```python
from build123d import *

# Parameters (mm, degrees)
SKETCH_1_W          = 10
SKETCH_1_H          = 12
SKETCH_1_W_2        = 5.2
SKETCH_1_H_2        = 5.2
EXTRUDE_1_DEPTH     = 4
SKETCH_2_R          = 0.6
CUT_EXTRUDE_1_DEPTH = 13.328828006
SKETCH_3_R          = 0.7
CUT_EXTRUDE_2_DEPTH = 14.601470509
SKETCH_3_3_R        = 1
CUT_EXTRUDE_3_DEPTH = 1.4
CUT_EXTRUDE_START   = -10.6
SKETCH_3_4_R        = 1
CUT_EXTRUDE_4_DEPTH = 1.4


with BuildPart() as part:
    # 草图1 → 凸台-拉伸1 (new body)
    with BuildSketch(Plane(origin=(0, 0, 0), x_dir=(1, 0, 0), z_dir=(0, 1, 0))):
        Rectangle(SKETCH_1_W, SKETCH_1_H)
        Rectangle(SKETCH_1_W_2, SKETCH_1_H_2, mode=Mode.SUBTRACT)
    extrude(amount=EXTRUDE_1_DEPTH)

    # 草图2 → 切除-拉伸1 (cut, through all)
    with BuildSketch(Plane(origin=(5, 0, 0), x_dir=(0, 0, -1), z_dir=(1, 0, 0))):
        with Locations((0, 2)):
            Circle(SKETCH_2_R)
    extrude(amount=-CUT_EXTRUDE_1_DEPTH, mode=Mode.SUBTRACT)

    # 草图3 → 切除-拉伸2 (cut, through all)
    with BuildSketch(Plane(origin=(0, 0, -6), x_dir=(-1, 0, 0), z_dir=(0, 0, -1))):
        with Locations((0, 2)):
            Circle(SKETCH_3_R)
    extrude(amount=-CUT_EXTRUDE_2_DEPTH, mode=Mode.SUBTRACT)

    # 草图3<3> → 切除-拉伸3 (cut)
    with BuildSketch(Plane(origin=(0, 0, -6), x_dir=(-1, 0, 0), z_dir=(0, 0, -1))):
        with Locations((0, 2)):
            Circle(SKETCH_3_3_R)
    extrude(amount=-CUT_EXTRUDE_3_DEPTH, mode=Mode.SUBTRACT)

    # 草图3<4> → 切除-拉伸4 (cut)
    with BuildSketch(Plane(origin=(0, 0, -6), x_dir=(-1, 0, 0), z_dir=(0, 0, -1)).offset(CUT_EXTRUDE_START)):
        with Locations((0, 2)):
            Circle(SKETCH_3_4_R)
    extrude(amount=-CUT_EXTRUDE_4_DEPTH, mode=Mode.SUBTRACT)


solid = part.part
```
Geometry: final body of the model. Coordinates: model frame, mm. A direction names the side the tool comes from. Coordinates: 2 decimals unless noted, no trailing zeros. Order: outer loops, then holes, each group sorted by start corner. A loop starts at its lowest first (then second) coordinate and runs counter-clockwise, first axis right, second up. Notation, with made-up numbers: (-18, 45) - (26, 45) arc R10 cw to (26, 53) - close; hole circle Ø11 at (-32, 17). An arc over 180 degrees is marked (long way). Return JSON: item names as keys, results as strings. Group by question number.
1. Cut plane C-C (z = 2). Output: boundary loops of the cut face in (x, y).
2. Pull-direction query (X, two-part tool) for faces 6 (the face through (-1.2, 2, -6)), 7 (the face through (-5, 1, 0)), 8 (the face through (-2.6, 2, 1)); classes: pulls with the +X half, pulls with the -X half, needs draft (parallel to the pull), parting line crosses it, or undercut.
3. Cut plane B-B (x = 0). Output: boundary loops of the cut face in (y, z).
4. Pin query (flat end, axial travel): pin 1 (1.6 mm diameter, centred on x = 0, y = 2, fed in from -Z); pin 2 (6 mm diameter, centred on x = 0.5, z = -1, fed in from +Y); pin 3 (1 mm diameter, centred on y = 2, z = 0, fed in from +X); pin 4 (1.6 mm diameter, centred on x = 0, y = 2, fed in from +Z). Return the tip coordinate at first contact, or that it passes through.
5. Cut plane A-A (y = 2). Count the separate pieces of the cut face and the enclosed holes in it, plus the area to 3 significant figures.
6. Cut plane D-D (x = -1.25). Output: boundary loops of the cut face in (y, z), plus the area to 3 significant figures.
7. Material intervals for line 1 along X through (y, z) = (0.45, -0.75); line 2 along Z through (x, y) = (-2.25, 0.3); line 3 along Z through (x, y) = (-3.25, 2.15), sorted ascending. Write a range as [from, to].
8. Set-up query: faces 1 (the face through (-1, 2, 2.6)), 2 (the face through (0, 1, -5)), 3 (the face through (0, 4, -3)), 4 (the face through (0, 1, 5)), 5 (the face through (3.817, 2.506, -0.323)). Return all of +Z, -Z, +X, -X, +Y, -Y with unobstructed straight access to the full face (end or side cutting, diameter ignored); none if empty.
Resolved:
{
 "1": {"outline": "(-5, 0) - (-2.6, 0) - (-2.6, 4) - (-5, 4) - close; (2.6, 0) - (5, 0) - (5, 4) - (2.6, 4) - close"},
 "2": {"face 6": "needs draft", "face 7": "pulls with the -X half", "face 8": "undercut"},
 "3": {"outline": "(0, -6) - (1, -6) - (1, -4.6) - (1.3, -4.6) - (1.3, -2.6) - (0, -2.6) - close; (0, 2.6) - (1.3, 2.6) - (1.3, 4.6) - (1, 4.6) - (1, 6) - (0, 6) - close; (2.7, -4.6) - (3, -4.6) - (3, -6) - (4, -6) - (4, -2.6) - (2.7, -2.6) - close; (2.7, 2.6) - (4, 2.6) - (4, 6) - (3, 6) - (3, 4.6) - (2.7, 4.6) - close"},
 "4": {"pin 1": "stops at z = -4.6", "pin 2": "stops at y = 4", "pin 3": "passes through", "pin 4": "stops at z = 4.6"},
 "5": {"separate pieces": "4", "enclosed holes": "0", "area": "76.0 mm²"},
 "6": {"outline": "(0, -6) - (4, -6) - (4, -2.6) - (0, -2.6) - close; (0, 2.6) - (4, 2.6) - (4, 6) - (0, 6) - close", "area": "27.2 mm²"},
 "7": {"line 1": "x = [-5, -2.6], [2.6, 5]", "line 2": "z = [-6, -2.6], [2.6, 6]", "line 3": "z = [-6, -0.58], [0.58, 6]"},
 "8": {"face 1": "+Y, -Y", "face 2": "-Z", "face 3": "+Z, -Z, +X, -X, +Y", "face 4": "+Z", "face 5": "+X, -X"}
}
